Source: three-view drawing plus pictorial views. Frame: mm from the lowest corner of the part. Coordinates: 2 decimals unless noted, no trailing zeros. Write each loop counter-clockwise with the first axis right and the second up, starting at its lowest first coordinate (ties: lowest second). Pieces come first, ordered by that corner, then holes. Notation, with made-up numbers: (-17.75, -17.75) -> (-9.75, -17.75) arc R23 cw to (-9.75, 15.25) -> close; hole circle Ø9 at (21, 55). An arc over 180 degrees is marked (long way). One line per question, with ' | ' between items. Start each with the question number.
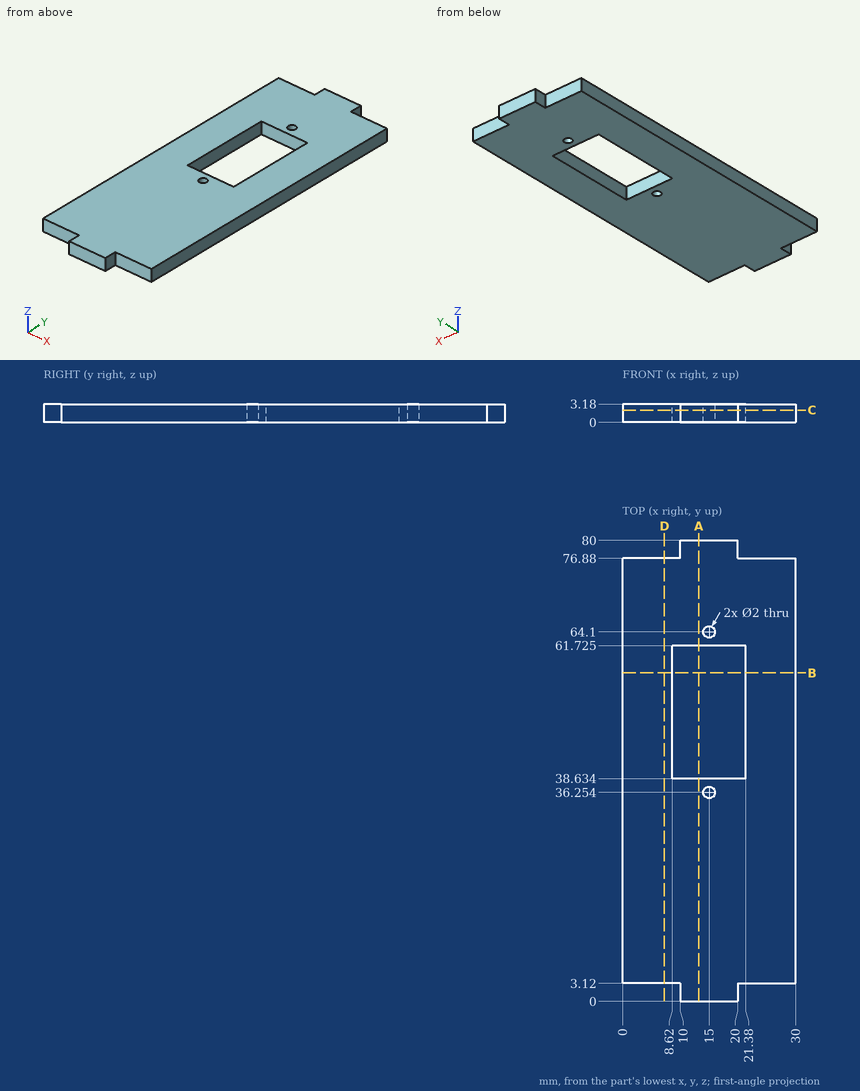
1) Section A-A, the plane x = 13.25. Return loops of the section in (y, z) (1 decimal).
2) First-contact query: P1, Ø1, axis at x = 22.5, z = 1.5, coming from the +Y side; P2, Ø1.6, axis at y = 78, z = 2, coming from the -X side; P3, Ø1.6, axis at x = 22.5, z = 1, coming from the -Y side; P4, Ø1.8, axis at x = 15, y = 36.25, coming from the -Z side. Flat tips, straight axial feed; report the tip coordinate or a pass-through.
3) Section B-B, the plane y = 57. Return loops of the section in (x, z).
4) Ray query, line 1 (Y direction, x = 15, z = 2.05) (1 decimal); line 2 (X direction, y = 39.5, z = 0.6); line 3 (Y direction, x = 17.25, z = 2.4) (1 decimal). Return the intervals inside material, ascending.
5) Section C-C, the plane z = 2.1. Return loops of the section in (x, y) (1 decimal), then the cut area to 3 significant figures.
6) Section D-D, the plane x = 7.25. Return loops of the section in (y, z).
Answer block:
1) outline: (0, 0) -> (38.6, 0) -> (38.6, 3.2) -> (0, 3.2) -> close; (61.7, 0) -> (80, 0) -> (80, 3.2) -> (61.7, 3.2) -> close
2) P1: stops at y = 76.88 | P2: stops at x = 10 | P3: stops at y = 3.12 | P4: passes through
3) outline: (0, 0) -> (8.62, 0) -> (8.62, 3.18) -> (0, 3.18) -> close; (21.38, 0) -> (30, 0) -> (30, 3.18) -> (21.38, 3.18) -> close
4) line 1: y = 0 to 35.3, 37.3 to 38.6, 61.7 to 63.1, 65.1 to 80 | line 2: x = 0 to 8.62, 21.38 to 30 | line 3: y = 0 to 38.6, 61.7 to 80
5) outline: (0, 3.1) -> (10, 3.1) -> (10, 0) -> (20, 0) -> (20, 3.1) -> (30, 3.1) -> (30, 76.9) -> (20, 76.9) -> (20, 80) -> (10, 80) -> (10, 76.9) -> (0, 76.9) -> close; hole (8.6, 38.6) -> (21.4, 38.6) -> (21.4, 61.7) -> (8.6, 61.7) -> close; hole circle Ø2 at (15, 36.3); hole circle Ø2 at (15, 64.1) | area: 1,970 mm2
6) outline: (3.12, 0) -> (76.88, 0) -> (76.88, 3.18) -> (3.12, 3.18) -> close
